Source: CAD feature listing. Evaluate the final solid. Frame: model axes, mm. Face numbers are marked on the shaded views. Coordinates: 2 decimals unless noted, no trailing zeros. Loops run counter-clockwise (first coordinate to the right, second up) from the corner with the lowest first, then second, coordinate; pieces in that order, holes last.
Item 1: Pin query (flat end, axial travel): pin 1 Ø5 at (x, y) = (-2, -0.5) entering from -Z; pin 2 Ø5 at (x, z) = (-3, -30) entering from +Y; pin 3 Ø1 at (x, z) = (-4.5, -86) entering from -Y. Return the tip coordinate at first contact, or that it passes through.
Item 2: Section query B-B, the plane z = 10.5. Return the cut outline in (x, y), then the cut area to 3 significant figures.
Item 3: Line query: probe 1 along Y at (x, z) = (8.55, 10.5); probe 2 along Z at (x, y) = (0, -11.8); probe 3 along Z at (x, y) = (7.4, 0). Output: solid intervals per line, ascending.
Item 4: Section query D-D, the plane z = -70. Return the cut outline in (x, y).
Item 5: Section query A-A, the plane z = -145. Return the cut outline in (x, y), then the cut area to 3 significant figures.
Item 6: Pull-direction query (Y, two-part tool) for the marked faces 1, 2, 3 and 4; classes: +Y half, -Y half, draft (parallel to the pull), parting line (faces both ways), or undercut.
Item 7: Section query C-C, the plane y = 8. Return the cut outline in (x, z), then the cut area to 3 significant figures.
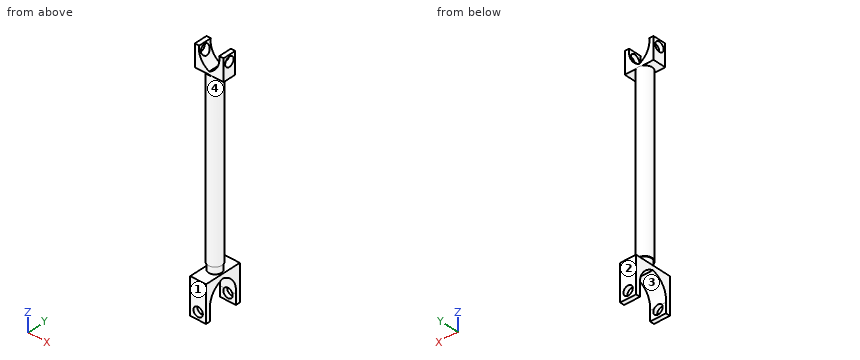
Autodesk Inventor part; units mm, degrees
ref_plane "YZ Plane" through (0, 0, 0) normal (1, 0, 0) x (0, 1, 0)
ref_plane "XZ Plane" through (0, 0, 0) normal (0, 1, 0) x (-1, 0, 0)
ref_plane "XY Plane" through (0, 0, 0) normal (0, 0, 1) x (1, 0, 0)
sketch "Sketch1" plane through (0, 0, 0) normal (0, 0, 1) x (1, 0, 0)
  circle A0 centre (0, 0) radius 5
  dimension "d0" = 10
extrude "Extrusion1" add sketch "Sketch1" against normal blind 120
sketch "Sketch2" plane through (0, 0, -120) normal (0, 0, -1) x (-1, 0, 0)
  circle A0 centre (0, 0) radius 4.5
  dimension "d3" = 9
extrude "Extrusion2" add sketch "Sketch2" along normal blind 5
sketch "Sketch3" plane through (0, 0, 0) normal (0, 0, 1) x (1, 0, 0)
  circle A0 centre (0, 0) radius 5
  line L0 (0, 0) -> (10, 0)
  line L1 (10, 0) -> (-10, 0)
  line L2 (0, 0) -> (0, 4.5)
  line L3 (0, 4.5) -> (0, -4.5)
  line L4 (0, -4.5) -> (-10, -4.5)
  line L5 (-10, -4.5) -> (-10, 0)
  line L6 (-10, 0) -> (-10, 4.5)
  line L7 (-10, 4.5) -> (0, 4.5)
  line L8 (0, 4.5) -> (10, 4.5)
  line L9 (10, 4.5) -> (10, -4.5)
  line L10 (10, -4.5) -> (0, -4.5)
  dimension "d8" = 4.5
  dimension "d53" = 4.5
  dimension "d56" = 20
  dimension "d57" = 10
  dimension "d58" = 10
extrude "Extrusion3" add sketch "Sketch3" along normal blind 15 contours L0 L2 L8 A0 | L0 L9 L10 A0 | A0 L10 L3 L0 | A0 L8 L9 L0 | L3 L4 A0 L1 | L1 A0 L7 L2 | A0 L1 L6 L7 | L4 L5 L1 A0
sketch "Sketch4" plane through (-10, -4.5, 0) normal (0, -1, 0) x (1, 0, 0)
  line L0 (0, 0) -> (7.8206, 0)
  line L1 (12.1794, 0) -> (7.8206, 0)
  line L2 (12.1794, 0) -> (20, 0)
  line L3 (20, 0) -> (20, 15)
  line L4 (0, 15) -> (20, 15)
  line L5 (0, 0) -> (0, 15)
  line L6 (10, 0) -> (10, 2)
  line L7 (0, 15) -> (20, 15)
  line L8 (0, 15) -> (3, 15)
  line L9 (20, 15) -> (17, 15)
  arc A0 (3, 15) -> (10, 2) centre (15.2365, 13.2043) ccw
  line L10 (10, 2) -> (10, 15)
  line L11 (4.3472, 7.3408) -> (0, 7.3408)
  line L12 (0, 0) -> (0, 15)
  line L13 (4.3472, 7.3408) -> (4.3472, 0)
  line L14 (15.6528, 7.3408) -> (20, 7.3408)
  line L15 (15.6528, 7.3408) -> (15.6528, 0)
  arc A1 (10, 2) -> (17, 15) centre (4.7635, 13.2043) ccw
  dimension "d12" = 2
  dimension "d13" = 3
  dimension "d14" = 3
extrude "Extrusion4" cut sketch "Sketch4" against normal blind 15 contours A0 L4 L10 | L10 L4 A1
sketch "Sketch5" plane through (10, -4.5, 0) normal (1, 0, 0) x (0, 0, -1)
  line L0 (0, 0) -> (0, 9)
  line L1 (0, 9) -> (-15, 9)
  line L2 (-15, 0) -> (-15, 9)
  line L3 (0, 0) -> (-15, 0)
  line L4 (-15, 0) -> (-15, 9)
  line L5 (-15, 4.5) -> (-10.5, 4.5)
  line L6 (0, 9) -> (0, 0)
  circle A0 centre (-10.5, 4.5) radius 3.25
  point P0 (0, 4.5)
  dimension "d19" = 4.5
  dimension "d55" = 6.5
extrude "Extrusion5" cut sketch "Sketch5" against normal blind 37.25 contours A0
sketch "Sketch6" plane through (0, 0, -125) normal (0, 0, -1) x (-1, 0, 0)
  circle A0 centre (0, 0) radius 4.5
  line L0 (0, 0) -> (0, 13)
  line L1 (0, -4.5) -> (0, 4.5)
  line L2 (0, 13) -> (0, -13)
  line L3 (0, -13) -> (-5.5, -13)
  line L4 (-5.5, -13) -> (5.5, -13)
  line L5 (5.5, -13) -> (5.5, 13)
  line L6 (5.5, 13) -> (-5.5, 13)
  line L7 (-5.5, 13) -> (-5.5, -13)
  dimension "d23" = 13
  dimension "d24" = 26
  dimension "d25" = 5.5
  dimension "d26" = 11
extrude "Extrusion6" add sketch "Sketch6" along normal blind 25
sketch "Sketch7" plane through (5.5, -13, -125) normal (1, 0, 0) x (0, 0, -1)
  line L0 (0, 26) -> (0, 0)
  line L1 (0, 0) -> (25, 0)
  line L2 (25, 26) -> (25, 0)
  line L3 (0, 26) -> (25, 26)
  line L4 (25, 26) -> (25, 0)
  line L5 (25, 26) -> (25, 23)
  line L6 (25, 0) -> (25, 3)
  line L7 (25, 23) -> (18, 23)
  line L8 (0, 8.5) -> (0, 17.5)
  line L9 (0, 13) -> (3, 13)
  arc A0 (18, 23) -> (3, 13) centre (16.2622, 9.3566) ccw
  line L10 (25, 3) -> (18, 3)
  line L11 (18, 3) -> (18, 23)
  arc A1 (3, 13) -> (18, 3) centre (16.3321, 16.7481) ccw
  point P0 (-125, 13)
  dimension "d29" = 3
  dimension "d30" = 3
  dimension "d32" = 7
  dimension "d33" = 3
extrude "Extrusion7" cut sketch "Sketch7" against normal blind 25 contours L2 L10 L11 L7 | A0 L11 A1
sketch "Sketch8" plane through (-5.5, 13, -125) normal (0, 1, 0) x (1, 0, 0)
  line L0 (0, 0) -> (11, 0)
  line L1 (11, 0) -> (11, 25)
  line L2 (0, 25) -> (11, 25)
  line L3 (0, 0) -> (0, 25)
  line L4 (5.5, 25) -> (5.5, 20)
  circle A0 centre (5.5, 20) radius 3.25
  line L5 (2.25, 20) -> (0, 20)
  line L6 (0, 18) -> (0, 25)
  line L7 (8.75, 20) -> (11, 20)
  line L8 (11, 25) -> (11, 18)
  point P0 (5.5, -125)
  dimension "d36" = 5
  dimension "d54" = 6.5
extrude "Extrusion8" cut sketch "Sketch8" against normal blind 30 contours A0
Verdict:
1. pin 1: stops at z = -129.24
1. pin 2: stops at y = 4.97
1. pin 3: stops at y = -3
2. outline: (-10, -4.5) - (-6.83, -4.5) - (-6.83, -3.25) - (-10, -3.25) - close; (-10, 3.25) - (-6.83, 3.25) - (-6.83, 4.5) - (-10, 4.5) - close; (6.83, -4.5) - (10, -4.5) - (10, -3.25) - (6.83, -3.25) - close; (6.83, 3.25) - (10, 3.25) - (10, 4.5) - (6.83, 4.5) - close
2. area: 15.8 mm2
3. probe 1: y = -4.5 to -3.25, 3.25 to 4.5
3. probe 2: z = -150 to -148.25, -141.75 to -125
3. probe 3: z = 0 to 7.25, 13.75 to 15
4. outline: circle Ø10 at (0, 0)
5. outline: (-5.5, -13) - (-3.25, -13) - (-3.25, -10) - (-5.5, -10) - close; (-5.5, 10) - (-3.25, 10) - (-3.25, 13) - (-5.5, 13) - close; (3.25, -13) - (5.5, -13) - (5.5, -10) - (3.25, -10) - close; (3.25, 10) - (5.5, 10) - (5.5, 13) - (3.25, 13) - close
5. area: 27.0 mm2
6. face 1: -Y half
6. face 2: +Y half
6. face 3: undercut
6. face 4: parting line
7. outline: (-5.5, -133.94) - (5.5, -133.94) - (5.5, -125) - (-5.5, -125) - close
7. area: 98.4 mm2
